For this review, take the finished solid that the model builds, in its own axes (mm). Face numbers are marked on the shaded views. A direction names the side the tool comes from. Give positions to 0.01 mm unless a question says otherwise; leave off trailing zeros. Write each loop counter-clockwise with the first axis right and the second up, starting at its lowest first coordinate (ties: lowest second). Pieces come first, ordered by that corner, then holes.
from build123d import *

# Parameters (mm, degrees)
SKETCH1_W                 = 41.656
SKETCH1_H                 = 45.847
BOSS_EXTRUDE1_DEPTH       = 25.4
SKETCH2_R                 = 16.129
CUT_EXTRUDE1_DEPTH        = 25.4
CUT_EXTRUDE2_DEPTH        = 3.81
CUT_EXTRUDE6_START        = -25.4
CUT_EXTRUDE6_DEPTH        = 25.4
CUT_EXTRUDE7_REACH        = 58.4
CUT_EXTRUDE7_END_RADIUS   = 16.129
SKETCH7_R                 = 3.048
SKETCH14_W                = 2.524584731
SKETCH14_H                = 21.209
SKETCH14_W_2              = 2.54
SKETCH14_W_3              = 7.43654476
SKETCH14_H_2              = 2.672753785
CUT_EXTRUDE10_DEPTH       = 2.54
SKETCH17_W                = 45.847
SKETCH17_H                = 22.86
BOSS_EXTRUDE3_DEPTH       = 3.175
CUT_EXTRUDE12_REACH       = 43.576
SKETCH12_R                = 3.048
SKETCH18_W                = 44.831
SKETCH18_H                = 22.86
BOSS_EXTRUDE4_DEPTH       = 1.5875
CUT_EXTRUDE13_DEPTH       = 44.190833792
CUT_EXTRUDE13_DEPTH_BACK  = 44.190833792
SKETCH11_R                = 3.048
SKETCH4_R                 = 1.778
CUT_EXTRUDE14_DEPTH       = 43.685983001
SKETCH19_R                = 3.175
SKETCH19_R_2              = 2.54
BOSS_EXTRUDE5_DEPTH       = 7.112
CIRPATTERN3_START         = 14.321246389
CIRPATTERN3_OUTLINE_R     = 3.048
CIRPATTERN3_OUTLINE_R_2   = 2.54
CIRPATTERN3_DEPTH         = 7.112
CIRPATTERN3_START_2       = 17.188786362
CIRPATTERN3_2_OUTLINE_R   = 3.048
CIRPATTERN3_2_OUTLINE_R_2 = 2.54
CIRPATTERN3_2_DEPTH       = 7.112
CIRPATTERN3_START_3       = 14.033500302
CIRPATTERN3_3_OUTLINE_W   = 10
CIRPATTERN3_3_OUTLINE_H   = 10
CIRPATTERN3_3_OUTLINE_R   = 2.54
CIRPATTERN3_3_DEPTH       = 7.112
SKETCH20_W                = 1.508584731
SKETCH20_H                = 6.858
SKETCH20_W_2              = 0.746584731
SKETCH20_H_2              = 8.128
BOSS_EXTRUDE6_DEPTH       = 2.54
SKETCH20_5_W              = 7.43654476
SKETCH20_5_H              = 2.672753785
CUT_EXTRUDE17_DEPTH       = 2.54
SKETCH21_W                = 3.175
SKETCH21_H                = 7.62
CUT_EXTRUDE18_DEPTH       = 1.27
CUT_EXTRUDE19_DEPTH       = 22.86


# Read off the part's stored shape, not the designer's step: CirPattern3
with BuildPart() as part:
    # Sketch1 → Boss-Extrude1 (new body)
    with BuildSketch(Plane(origin=(0, 0, 0), x_dir=(1, 0, 0), z_dir=(0, 1, 0))):
        Rectangle(SKETCH1_W, SKETCH1_H)
    extrude(amount=BOSS_EXTRUDE1_DEPTH)

    # Sketch2 → Cut-Extrude1 (cut)
    with BuildSketch(Plane(origin=(0, 25.4, 0), x_dir=(1, 0, 0), z_dir=(0, 1, 0))):
        with Locations(Location((0, 2.0955, 0), (0, 0, 270))):
            Circle(SKETCH2_R)
    extrude(amount=-CUT_EXTRUDE1_DEPTH, mode=Mode.SUBTRACT)

    # Sketch3 → Cut-Extrude2 (cut)
    with BuildSketch(Plane(origin=(0, 25.4, 0), x_dir=(1, 0, 0), z_dir=(0, 1, 0))):
        Polygon((17.018, -1.7145), (19.812, -1.7145), (20.828, -1.7145), (20.828, 5.9055), (17.018, 5.9055), align=None)
        Polygon((-17.018, 5.9055), (-19.812, 5.9055), (-20.828, 5.9055), (-20.828, -1.7145), (-19.812, -1.7145), (-17.018, -1.7145), align=None)
    extrude(amount=-CUT_EXTRUDE2_DEPTH, mode=Mode.SUBTRACT)

    # Sketch6 → Cut-Extrude6 (cut)
    with BuildSketch(Plane(origin=(0, 25.4, 0), x_dir=(1, 0, 0), z_dir=(0, 1, 0)).offset(CUT_EXTRUDE6_START)):
        with BuildLine():
            ThreePointArc((-2.800771458, 17.979464248), (-1.405734975, 18.163124286), (0, 18.2245))
            ThreePointArc((0, 18.2245), (1.405734975, 18.163124286), (2.800771458, 17.979464248))
            Line((2.800771458, 17.979464248), (2.955144688, 18.854958341))
            ThreePointArc((2.955144688, 18.854958341), (0, 19.1135), (-2.955144688, 18.854958341))
            Line((-2.955144688, 18.854958341), (-2.800771458, 17.979464248))
        make_face()
        with BuildLine():
            Line((0, 18.2245), (0, 2.0955))
            Line((0, 2.0955), (2.800771458, 17.979464248))
            ThreePointArc((2.800771458, 17.979464248), (1.405734975, 18.163124286), (0, 18.2245))
        make_face()
        with BuildLine():
            Line((-2.800771458, 17.979464248), (0, 2.0955))
            Line((0, 2.0955), (0, 18.2245))
            ThreePointArc((0, 18.2245), (-1.405734975, 18.163124286), (-2.800771458, 17.979464248))
        make_face()
    extrude(amount=CUT_EXTRUDE6_DEPTH, mode=Mode.SUBTRACT)

    # Cut-Extrude7: up to this cylinder (the profile starts outside it)
    cut_extrude7_end = Plane(origin=(0, 16.002, -2.0955), z_dir=(0, 1, 0)) * Cylinder(CUT_EXTRUDE7_END_RADIUS, 150.058, mode=Mode.PRIVATE)
    # Sketch7 → Cut-Extrude7 (cut, up to the surface)
    with BuildSketch(Plane.XY.offset(22.9235), mode=Mode.PRIVATE) as cut_extrude7_sk1:
        with Locations((0, 16.002)):
            Circle(SKETCH7_R)
    cut_extrude7_tool1 = extrude(cut_extrude7_sk1.sketch, amount=-CUT_EXTRUDE7_REACH, mode=Mode.PRIVATE) - cut_extrude7_end
    add(cut_extrude7_tool1.solids().sort_by_distance((0, 16.002, 22.9235))[0], mode=Mode.SUBTRACT)

    # Sketch14 → Cut-Extrude10 (cut)
    with BuildSketch(Plane(origin=(0, 25.4, 0), x_dir=(1, 0, 0), z_dir=(0, 1, 0))):
        Polygon((20.828, 22.9235), (-20.828, 22.9235), (-20.828, 5.9055), (-18.303415269, 5.9055), (-18.303415269, 20.3835), (20.828, 20.3835), align=None)
        with Locations((-19.565707635, -12.319)):
            Rectangle(SKETCH14_W, SKETCH14_H)
        with Locations((19.558, -12.319)):
            Rectangle(SKETCH14_W_2, SKETCH14_H)
        with Locations((0, -20.25731759)):
            Rectangle(SKETCH14_W_3, SKETCH14_H_2)
    extrude(amount=-CUT_EXTRUDE10_DEPTH, mode=Mode.SUBTRACT)

    # Sketch17 → Boss-Extrude3 (add)
    with BuildSketch(Plane(origin=(20.828, 0, 0), x_dir=(0, 0, -1), z_dir=(1, 0, 0))):
        with Locations((0, 11.43)):
            Rectangle(SKETCH17_W, SKETCH17_H)
    extrude(amount=BOSS_EXTRUDE3_DEPTH)

    # Cut-Extrude12: up to this plane
    cut_extrude12_end = Plane(origin=(24.003, 0, 0), z_dir=(1, 0, 0))
    # Sketch12 → Cut-Extrude12 (cut, up to the surface)
    with BuildSketch(Plane(origin=(0.914260378, 0, -0.535980498), x_dir=(-0.50574390925612, 0, -0.862683660590797), z_dir=(0.862683660590797, 0, -0.50574390925612)), mode=Mode.PRIVATE) as cut_extrude12_sk1:
        with Locations(Location((1.807753611, 16.002, 0), (0, 0, 180))):
            Circle(SKETCH12_R)
    cut_extrude12_tool1 = split(extrude(cut_extrude12_sk1.sketch, amount=CUT_EXTRUDE12_REACH, mode=Mode.PRIVATE), bisect_by=cut_extrude12_end, keep=Keep.BOTH, mode=Mode.PRIVATE)
    add(cut_extrude12_tool1.solids().sort_by_distance((0, 16.002, -2.0955))[0], mode=Mode.SUBTRACT)

    # Sketch18 → Boss-Extrude4 (add)
    with BuildSketch(Plane(origin=(0, 0, -22.9235), x_dir=(-1, 0, 0), z_dir=(0, 0, -1))):
        with Locations((-1.5875, 11.43)):
            Rectangle(SKETCH18_W, SKETCH18_H)
    extrude(amount=BOSS_EXTRUDE4_DEPTH)

    # Sketch11 → Cut-Extrude13 (cut, two sides: drawn at the far end of the back side and taken through both)
    with BuildSketch(Plane(origin=(-0.914260378, 0, -1.559519502), x_dir=(0.862683660590797, 0, -0.50574390925612), z_dir=(0.50574390925612, 0, 0.862683660590797)).offset(-CUT_EXTRUDE13_DEPTH_BACK)):
        with Locations((1.059786362, 16.002)):
            Circle(SKETCH11_R)
    extrude(amount=CUT_EXTRUDE13_DEPTH + CUT_EXTRUDE13_DEPTH_BACK, mode=Mode.SUBTRACT)

    # Sketch4 → Cut-Extrude14 (cut, through all)
    with BuildSketch(Plane(origin=(0, 25.4, 0), x_dir=(1, 0, 0), z_dir=(0, 1, 0))):
        with Locations(Location((-16.002, -13.9065, 0), (0, 0, 270))):
            Circle(SKETCH4_R)
        with Locations(Location((-16.002, 18.0975, 0), (0, 0, 90))):
            Circle(SKETCH4_R)
        with Locations(Location((16.002, 18.0975, 0), (0, 0, 270))):
            Circle(SKETCH4_R)
        with Locations(Location((16.002, -13.9065, 0), (0, 0, 90))):
            Circle(SKETCH4_R)
    extrude(amount=-CUT_EXTRUDE14_DEPTH, mode=Mode.SUBTRACT)

    # Sketch19 → Boss-Extrude5 (add)
    with BuildSketch(Plane(origin=(-9.07140389, 0, -15.473744264), x_dir=(0.8626836605907969, 0, -0.5057439092561202), z_dir=(0.5057439092561202, 0, 0.8626836605907969))):
        with Locations((1.059786362, 16.002)):
            Circle(SKETCH19_R)
        with Locations((1.059786362, 16.002)):
            Circle(SKETCH19_R_2, mode=Mode.SUBTRACT)
    extrude(amount=-BOSS_EXTRUDE5_DEPTH)

    # CirPattern3 outline → CirPattern3 (add)
    with BuildSketch(Plane(origin=(0, 0, 0), x_dir=(0.8626836605907969, 0, -0.5057439092561199), z_dir=(0.50574390925612, 0, 0.862683660590797)).offset(CIRPATTERN3_START)):
        with Locations((1.059786362, 16.002)):
            Circle(CIRPATTERN3_OUTLINE_R)
        with Locations((1.059786362, 16.002)):
            Circle(CIRPATTERN3_OUTLINE_R_2, mode=Mode.SUBTRACT)
    extrude(amount=CIRPATTERN3_DEPTH)

    # CirPattern3 2 outline → CirPattern3 2 (add)
    with BuildSketch(Plane(origin=(0, 0, 0), x_dir=(0.5057439092561169, 0, 0.8626836605907988), z_dir=(0.8626836605907988, 0, -0.5057439092561169)).offset(CIRPATTERN3_START_2)):
        with Locations((-1.807753611, -16.002)):
            Circle(CIRPATTERN3_2_OUTLINE_R)
        with Locations((-1.807753611, -16.002)):
            Circle(CIRPATTERN3_2_OUTLINE_R_2, mode=Mode.SUBTRACT)
    extrude(amount=CIRPATTERN3_2_DEPTH)

    # CirPattern3 3 outline → CirPattern3 3 (add)
    with BuildSketch(Plane(origin=(0, 0, 0), x_dir=(0.9999998560090501, 0, -0.0005366394310553081), z_dir=(0.0005366394310553081, 0, 0.9999998560090502)).offset(CIRPATTERN3_START_3)):
        with Locations((0, 16)):
            Rectangle(CIRPATTERN3_3_OUTLINE_W, CIRPATTERN3_3_OUTLINE_H)
        with Locations((0.001124528, 16.002)):
            Circle(CIRPATTERN3_3_OUTLINE_R, mode=Mode.SUBTRACT)
    extrude(amount=CIRPATTERN3_3_DEPTH)

    # Sketch20 → Boss-Extrude6 (add)
    with BuildSketch(Plane(origin=(0, 25.4, 0), x_dir=(1, 0, 0), z_dir=(0, 1, 0))):
        Polygon((9.835016705, 20.3835), (19.741016705, 20.3835), (19.741016705, 21.9075), (8.311016705, 21.9075), align=None)
        with Locations((-19.057707635, 16.7005)):
            Rectangle(SKETCH20_W, SKETCH20_H)
        Polygon((19.05, -6.5405), (18.288, -7.3025), (18.288, -16.9545), (19.05, -16.9545), align=None)
        with Locations((-18.676707635, -12.8905)):
            Rectangle(SKETCH20_W_2, SKETCH20_H_2)
    extrude(amount=-BOSS_EXTRUDE6_DEPTH)

    # Sketch20<5> → Cut-Extrude17 (cut)
    with BuildSketch(Plane(origin=(0, 25.4, 0), x_dir=(1, 0, 0), z_dir=(0, 1, 0))):
        Polygon((19.741016705, 20.3835), (19.741016705, 18.0975), (19.741016705, 10.4775), (9.835016705, 20.3835), (-18.303415269, 20.3835), (-18.303415269, 20.1295), (-16.002, 20.1295), (-9.906, 20.1295), (-16.764, 13.2715), (-18.303415269, 13.2715), (-18.303415269, 5.9055), (-17.018, 5.9055), (-17.018, -1.7145), (-18.303415269, -1.7145), (-18.303415269, -8.8265), (-17.018, -8.8265), (-12.7, -13.1445), (-12.7, -16.9545), (-16.002, -16.9545), (-18.303415269, -16.9545), (-18.303415269, -22.9235), (18.288, -22.9235), (18.288, -16.9545), (16.002, -16.9545), (9.652, -16.9545), (9.652, -15.9385), (18.288, -7.3025), (18.288, -1.7145), (17.018, -1.7145), (17.018, 5.9055), (20.828, 5.9055), (20.828, 20.3835), align=None)
        with Locations((0, -20.25731759)):
            Rectangle(SKETCH20_5_W, SKETCH20_5_H, mode=Mode.SUBTRACT)
        with BuildLine():
            ThreePointArc((2.800771458, 17.979464248), (0, -14.0335), (-2.800771458, 17.979464248))
            Line((-2.800771458, 17.979464248), (-2.955144688, 18.854958341))
            ThreePointArc((-2.955144688, 18.854958341), (0, 19.1135), (2.955144688, 18.854958341))
            Line((2.955144688, 18.854958341), (2.800771458, 17.979464248))
        make_face(mode=Mode.SUBTRACT)
    extrude(amount=-CUT_EXTRUDE17_DEPTH, mode=Mode.SUBTRACT)

    # Sketch21 → Cut-Extrude18 (cut)
    with BuildSketch(Plane(origin=(0, 22.86, 0), x_dir=(1, 0, 0), z_dir=(0, 1, 0))):
        with Locations((22.4155, 2.0955)):
            Rectangle(SKETCH21_W, SKETCH21_H)
    extrude(amount=-CUT_EXTRUDE18_DEPTH, mode=Mode.SUBTRACT)

    # Sketch22 → Cut-Extrude19 (cut)
    with BuildSketch(Plane(origin=(0, 22.86, 0), x_dir=(1, 0, 0), z_dir=(0, 1, 0))):
        with BuildLine():
            ThreePointArc((15.672540987, -1.7145), (0, -14.0335), (-15.672540987, -1.7145))
            Line((-15.672540987, -1.7145), (-16.906599333, -2.0145))
            ThreePointArc((-16.906599333, -2.0145), (-13.10543472, -9.348834048), (-6.35, -14.103348755))
            Line((-6.35, -14.103348755), (-6.35, -22.9235))
            Line((-6.35, -22.9235), (6.35, -22.9235))
            Line((6.35, -22.9235), (6.35, -14.103348755))
            ThreePointArc((6.35, -14.103348755), (13.10543472, -9.348834048), (16.906599333, -2.0145))
            Line((16.906599333, -2.0145), (15.672540987, -1.7145))
        make_face()
    extrude(amount=-CUT_EXTRUDE19_DEPTH, mode=Mode.SUBTRACT)


solid = part.part
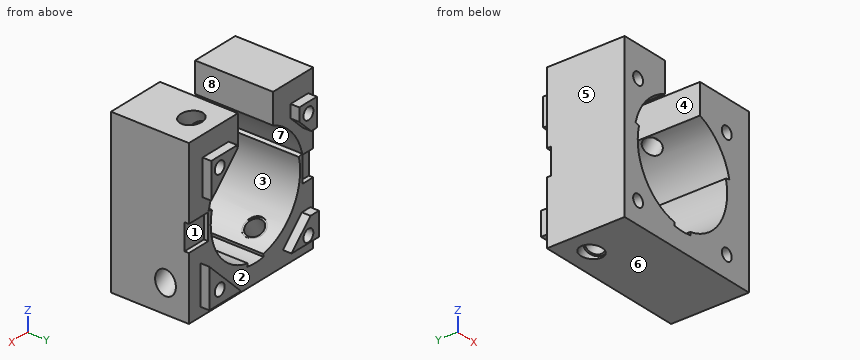
(1) We need section C-C (x = 1). Write out the cut boundary in (y, z), and give its area (3 significant figures).
(2) The part is to be moulded in two halves that separate along Z. For the marked faces 6, 7 and 8, say which applies: +Z half, -Z half, draft (parallel to the pull), parting line (faces both ways), or undercut.
(3) Clearance check with flat-ended pins moving along their axes: pin 1 Ø1 at (x, y) = (-17.5, 24.5) entering from -Z; pin 2 Ø5.5 at (x, z) = (-16, 13.91) entering from -Y; pin 3 Ø1.3 at (x, y) = (-16, 24) entering from +Z; pin 4 Ø1.4 at (y, z) = (22.5, -1) entering from +X. State where each tip first meets the part, or that it passes through.
(4) We need section A-A (z = 4.5). Write out the cut boundary in (x, y).
(5) We need section B-B (y = 9.25). Write out the cut boundary in (x, z).
(6) For L1, parallel to X at y = 9.25, z = 14.5; L2, parallel to Y at x = 21, z = 6.5; L3, parallel to X at y = 12, z = -2, list the stretches that pass through material, from the lowest coordinate up.
(7) Tool access review of the marked faces 1, 2, 3, 4 and 5: name each direction out of +Z, -Z, +X, -X, +Y, -Y from which nothing blocks a thin tool from reaching the whole face with its end or side.
(8) We need section D-D (x = -4.5). Write out the cut boundary in (y, z), and give its area (3 significant figures).
The answers:
1. outline: (0, -24.51) - (22.86, -24.51) - (22.86, -19.08) - (0, -19.08) - close
1. area: 124 mm2
2. face 6: -Z half
2. face 7: undercut
2. face 8: draft
3. pin 1: stops at z = -20.13
3. pin 2: stops at y = 0
3. pin 3: stops at z = 16.95
3. pin 4: stops at x = 17.02
4. outline: (-20.83, 0) - (-16.1, 0) - (-16.1, 22.86) - (-20.83, 22.86) - close; (16.1, 0) - (24, 0) - (24, 22.86) - (16.1, 22.86) - close
5. outline: (-20.83, -24.51) - (24, -24.51) - (24, 22.92) - (6.35, 22.92) - (6.35, 14.1) arc R17.4 cw to (16.91, 2.01) - (15.67, 1.71) arc R16.13 cw to (2.8, -17.98) - (2.96, -18.85) arc R17.02 cw to (-2.96, -18.85) - (-2.8, -17.98) arc R16.13 cw to (-15.67, 1.71) - (-16.91, 2.01) arc R17.4 cw to (-6.35, 14.1) - (-6.35, 22.92) - (-20.83, 22.92) - close; hole circle Ø3.56 at (-16, -18.1); hole circle Ø3.56 at (-16, 13.91); hole circle Ø3.56 at (16, -18.1); hole circle Ø3.56 at (16, 13.91)
6. L1: x = -20.83 to -17.68, -14.33 to -6.35, 6.35 to 14.33, 17.68 to 24
6. L2: y = 0 to 22.86
6. L3: x = -20.83 to -16.13, 16.13 to 24
7. face 1: +X, +Y
7. face 2: +Y
7. face 3: +Y, -Y
7. face 4: +Z, +Y, -Y
7. face 5: +Z, -Z, -X, +Y, -Y
8. outline: (0, -24.51) - (22.86, -24.51) - (22.86, -17.58) - (0, -17.58) - close
8. area: 158 mm2
